Work out the finished part from the listing and answer in its coordinate system (mm). A direction names the side the tool comes from. Coordinates: 2 decimals unless noted, no trailing zeros. Write each loop counter-clockwise with the first axis right and the second up, starting at its lowest first coordinate (ties: lowest second). Pieces come first, ordered by that corner, then holes. Notation, with made-up numbers: (-22.5, 41) - (0.5, 41) arc R26 ccw to (0.5, 72) - close; hole circle Ø11 at (13.25, -32.5). An arc over 180 degrees is marked (long way). Use one line per item in the form item = value. Start each with the question number.
Item 1: Consider probe 1 along Y at (x, z) = (-15.5, -2); probe 2 along Y at (x, z) = (7, 0); probe 3 along Z at (x, y) = (-1.5, -43). Determine where each line is inside the solid, lowest interval first.
Item 2: A cutting plane is placed at C-C (y = -3). Write down the section's boundary in (x, z).
Item 3: A cutting plane is placed at B-B (y = 6). Write down the section's boundary in (x, z).
Item 4: Given pin 1 (12 mm diameter, centred on y = 2.5, z = -5.5, fed in from -X); pin 2 (1.5 mm diameter, centred on y = 2.5, z = 6, fed in from -X); pin 3 (1 mm diameter, centred on x = -10.5, y = -25, fed in from -Z), each flat-ended and moving along its own axis, determine where each tip first touches the part or whether it passes through.
Item 5: For faces 1 (the flat face through (13, 0, -1)), 2 (the flat face through (14.37, 6.26, 8.45)), determine the directions among +Z, -Z, +X, -X, +Y, -Y from which every point of the face is accessible in a straight line to the end or side of a thin tool.
Item 6: A cutting plane is placed at A-A (x = 0). Write down the section's boundary in (y, z).
Item 7: A cutting plane is placed at D-D (x = -17). Write down the section's boundary in (y, z), then the cut area to 3 significant figures.
from build123d import *

# Parameters (mm, degrees)
BOSS_EXTRUDE1_DEPTH = 12.7
SKETCH2_R           = 12.7
BOSS_EXTRUDE2_DEPTH = 44.45
SKETCH3_R           = 12.7
BOSS_EXTRUDE3_DEPTH = 6.35
CHAMFER1_SIZE       = 6.35


with BuildPart() as part:
    # Sketch1 → Boss-Extrude1 (new body)
    with BuildSketch(Plane(origin=(0, 0, 0), x_dir=(1, 0, 0), z_dir=(0, 1, 0))):
        Polygon((19.247414599, 0), (9.6237073, 16.66875), (-9.6237073, 16.66875), (-19.247414599, 0), (-9.6237073, -16.66875), (9.6237073, -16.66875), align=None)
    extrude(amount=BOSS_EXTRUDE1_DEPTH)

    # Sketch2 → Boss-Extrude2 (add)
    with BuildSketch(Plane.XZ):
        with Locations(Location((0, 0, 0), (0, 0, 270))):
            Circle(SKETCH2_R)
    extrude(amount=BOSS_EXTRUDE2_DEPTH)

    # Sketch3 → Boss-Extrude3 (add)
    with BuildSketch(Plane(origin=(0, -44.45, 0), x_dir=(-1, 0, 0), z_dir=(0, -1, 0))):
        with Locations(Location((0, 0, 0), (0, 0, 90))):
            Circle(SKETCH3_R)
    extrude(amount=BOSS_EXTRUDE3_DEPTH)

    # Chamfer1
    chamfer1_edges = [part.edges().sort_by_distance(p)[0] for p in [
        (0, -50.8, 12.7),
    ]]
    chamfer(chamfer1_edges, length=CHAMFER1_SIZE)


solid = part.part
Answer:
q1.probe_1 = 0 to 12.7
q1.probe_2 = -50.15 to 12.7
q1.probe_3 = -12.61 to 12.61
q2.outline = circle Ø25.4 at (0, 0)
q3.outline = (-19.25, 0) - (-9.62, -16.67) - (9.62, -16.67) - (19.25, 0) - (9.62, 16.67) - (-9.62, 16.67) - close
q4.pin_1 = -19.25
q4.pin_2 = -16.22
q4.pin_3 = -7.83
q5.face_1 = -Y
q5.face_2 = +Z, +X, +Y, -Y
q6.outline = (-50.8, -6.35) - (-44.45, -12.7) - (0, -12.7) - (0, -16.67) - (12.7, -16.67) - (12.7, 16.67) - (0, 16.67) - (0, 12.7) - (-44.45, 12.7) - (-50.8, 6.35) - close
q7.outline = (0, -3.89) - (12.7, -3.89) - (12.7, 3.89) - (0, 3.89) - close
q7.area = 98.9 mm²
